Here's the drawing with two shaded views (mm, measured from the low corner). I have some questions. A direction names the side the tool comes from. Coordinates: 2 decimals unless noted, no trailing zeros. Write each loop counter-clockwise with the first axis right and the second up, starting at its lowest first coordinate (ties: lowest second). Pieces come first, ordered by that corner, then holes. Notation, with made-up numbers: (-30, -34) - (-2, -34) arc R32 cw to (-2, -8) - close; hole circle Ø3 at (27, -36.75). An arc over 180 degrees is marked (long way). Answer in a Markdown table with one row per item. Add a question column.
Item 1: Imagine slicing it at A-A (x = 17). Please give me the cut outline in (y, z), plus the area to 3 significant figures.
Item 2: Imagine slicing it at B-B (z = 25). Please give me the cut outline in (x, y).
Item 3: Imagine slicing it at C-C (y = 2.25). Please give me the cut outline in (x, z).
Item 4: Which directions (+Z, -Z, +X, -X, +Y, -Y) give clear straight access to the entire face, cutting with the end or side of a thin tool? Please do the marked faces 1 and 2.
Item 5: If I drill on probe 1 along Z at (x, y) = (7.5, 3.1); probe 2 along Z at (x, y) = (19.5, 0.9), over which ranges is the centre line in solid material (lowest first)? Write a range as from..to.
Item 6: I'm going to push a flat-ended pin straight in: pin 1 (2 mm diameter, centred on x = 17.5, z = 35, fed in from -Y). Where does the tip first touch, or does it pass through?
Item 7: We'd pull the mould along Z, two halves only. Please class the marked faces 3 and 4: +Z half, -Z half, draft (parallel to the pull), parting line (faces both ways), or undercut.
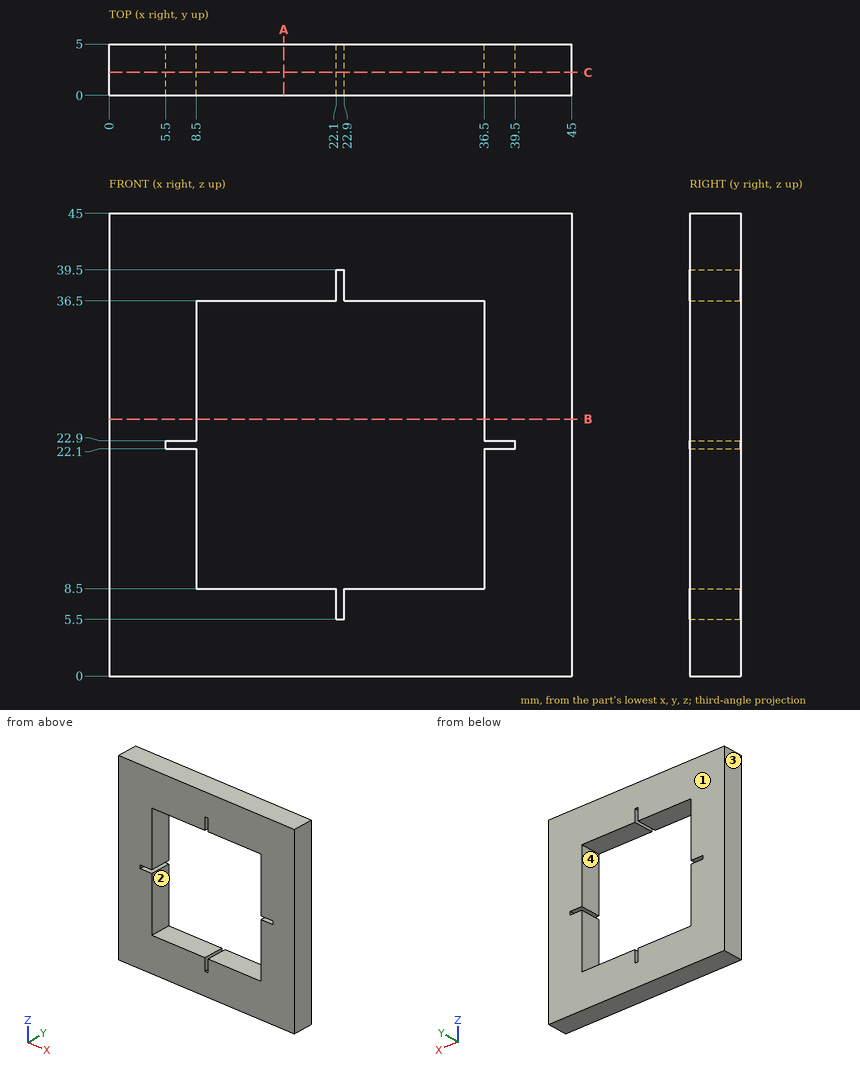
Here are the results:
| question | item | result |
|---|---|---|
| 1 | outline | (0, 0) - (5, 0) - (5, 8.5) - (0, 8.5) - close; (0, 36.5) - (5, 36.5) - (5, 45) - (0, 45) - close |
| 1 | area | 85.0 mm2 |
| 2 | outline | (0, 0) - (8.5, 0) - (8.5, 5) - (0, 5) - close; (36.5, 0) - (45, 0) - (45, 5) - (36.5, 5) - close |
| 3 | outline | (0, 0) - (45, 0) - (45, 45) - (0, 45) - close; hole (5.5, 22.1) - (8.5, 22.1) - (8.5, 8.5) - (22.1, 8.5) - (22.1, 5.5) - (22.9, 5.5) - (22.9, 8.5) - (36.5, 8.5) - (36.5, 22.1) - (39.5, 22.1) - (39.5, 22.9) - (36.5, 22.9) - (36.5, 36.5) - (22.9, 36.5) - (22.9, 39.5) - (22.1, 39.5) - (22.1, 36.5) - (8.5, 36.5) - (8.5, 22.9) - (5.5, 22.9) - close |
| 4 | face 1 | +Z, -Z, +X, -X, +Y |
| 4 | face 2 | +Y, -Y |
| 5 | probe 1 | z = 0..22.1, 22.9..45 |
| 5 | probe 2 | z = 0..8.5, 36.5..45 |
| 6 | pin 1 | passes through |
| 7 | face 3 | draft |
| 7 | face 4 | undercut |
